Check sheet for the modelled part. Datum: model origin and axes. Units: mm. A direction names the side the tool comes from. Coordinates: 2 decimals unless noted, no trailing zeros. Order: outer loops, then holes, each group sorted by start corner. A loop starts at its lowest first (then second) coordinate and runs counter-clockwise, first axis right, second up.
from build123d import *
from OCP.BRepFilletAPI import BRepFilletAPI_MakeChamfer

# Parameters (mm, degrees)
SCHIZZO1_R                   = 18.5
ESTRUSIONE_ESTRUSIONE1_DEPTH = 29.3
SCHIZZO2_R                   = 16.5
ESTRUSIONE_ESTRUSIONE2_DEPTH = 22.7
SCHIZZO3_R                   = 15.85
TAGLIO_ESTRUSIONE1_DEPTH     = 1.5
SCHIZZO4_R                   = 2.75
SCHIZZO4_R_2                 = 3.925
ESTRUSIONE_ESTRUSIONE3_DEPTH = 2
SCHIZZO5_W                   = 0.5
SCHIZZO5_H                   = 2.9
ESTRUSIONE_ESTRUSIONE4_DEPTH = 4.5
SMUSSO1_SIZE                 = 1
SMUSSO1_SIZE2                = 0.577350269
TAGLIO_ESTRUSIONE2_DEPTH     = 68.129073433
SCHIZZO7_R                   = 1.1
TAGLIO_ESTRUSIONE3_DEPTH     = 2
SCHIZZO8_R                   = 1
ESTRUSIONE_ESTRUSIONE5_DEPTH = 4.75
SCHIZZO9_R                   = 1.5
TAGLIO_ESTRUSIONE4_DEPTH     = 5
SCHIZZO10_R                  = 6
ESTRUSIONE_ESTRUSIONE6_DEPTH = 6
SCHIZZO11_R                  = 3
ESTRUSIONE_ESTRUSIONE7_DEPTH = 3.5
ESTRUSIONE_ESTRUSIONE8_DEPTH = 12
CROQUIS1_R                   = 2
CORTAR_EXTRUIR1_DEPTH        = 10


with BuildPart() as part:
    # Schizzo1 → Estrusione-Estrusione1 (new body)
    with BuildSketch(Plane(origin=(0, 0, 0), x_dir=(1, 0, 0), z_dir=(0, 1, 0))):
        with Locations(Location((0, 0, 0), (0, 0, 270))):
            Circle(SCHIZZO1_R)
    extrude(amount=ESTRUSIONE_ESTRUSIONE1_DEPTH)

    # Schizzo2 → Estrusione-Estrusione2 (add)
    with BuildSketch(Plane(origin=(0, 29.3, 0), x_dir=(1, 0, 0), z_dir=(0, 1, 0))):
        with Locations(Location((0, 0, 0), (0, 0, 270))):
            Circle(SCHIZZO2_R)
    extrude(amount=ESTRUSIONE_ESTRUSIONE2_DEPTH)

    # Schizzo3 → Taglio-Estrusione1 (cut)
    with BuildSketch(Plane(origin=(0, 52, 0), x_dir=(1, 0, 0), z_dir=(0, 1, 0))):
        with Locations(Location((0, 0, 0), (0, 0, 270))):
            Circle(SCHIZZO3_R)
    extrude(amount=-TAGLIO_ESTRUSIONE1_DEPTH, mode=Mode.SUBTRACT)

    # Schizzo4 → Estrusione-Estrusione3 (add)
    with BuildSketch(Plane(origin=(0, 50.5, 0), x_dir=(1, 0, 0), z_dir=(0, 1, 0))):
        with Locations(Location((11.5, 0, 0), (0, 0, 270))):
            Circle(SCHIZZO4_R)
        with Locations(Location((-11.5, 0, 0), (0, 0, 270))):
            Circle(SCHIZZO4_R)
        with Locations(Location((0, 0, 0), (0, 0, 270))):
            Circle(SCHIZZO4_R_2)
    extrude(amount=ESTRUSIONE_ESTRUSIONE3_DEPTH)

    # Schizzo5 → Estrusione-Estrusione4 (add)
    with BuildSketch(Plane(origin=(0, 52.5, 0), x_dir=(1, 0, 0), z_dir=(0, 1, 0))):
        with Locations((-11.5, 0)):
            Rectangle(SCHIZZO5_W, SCHIZZO5_H)
        with Locations((11.5, 0)):
            Rectangle(SCHIZZO5_W, SCHIZZO5_H)
    extrude(amount=ESTRUSIONE_ESTRUSIONE4_DEPTH)

    # Smusso1: one chamfer whose edges measure the first distance from different faces: ONE call of the kernel's chamfer builder (chamfer() names one face for all edges)
    smusso1_edges_1 = [part.edges().sort_by_distance(p)[0] for p in [
        (-11.5, 57, -1.45),
    ]]
    smusso1_side_1 = [part.faces().sort_by_distance(p)[0] for p in [
        (-11.5, 54.75, -1.45),
    ]]
    smusso1_edges_2 = [part.edges().sort_by_distance(p)[0] for p in [
        (-11.5, 57, 1.45),
    ]]
    smusso1_side_2 = [part.faces().sort_by_distance(p)[0] for p in [
        (-11.5, 54.75, 1.45),
    ]]
    smusso1_edges_3 = [part.edges().sort_by_distance(p)[0] for p in [
        (11.5, 57, -1.45),
    ]]
    smusso1_side_3 = [part.faces().sort_by_distance(p)[0] for p in [
        (11.5, 54.75, -1.45),
    ]]
    smusso1_edges_4 = [part.edges().sort_by_distance(p)[0] for p in [
        (11.5, 57, 1.45),
    ]]
    smusso1_side_4 = [part.faces().sort_by_distance(p)[0] for p in [
        (11.5, 54.75, 1.45),
    ]]
    smusso1 = BRepFilletAPI_MakeChamfer(part.part.solid().wrapped)
    for e in smusso1_edges_1:
        smusso1.Add(SMUSSO1_SIZE, SMUSSO1_SIZE2, e.wrapped, smusso1_side_1[0].wrapped)  # the first distance lies on this face
    for e in smusso1_edges_2:
        smusso1.Add(SMUSSO1_SIZE, SMUSSO1_SIZE2, e.wrapped, smusso1_side_2[0].wrapped)  # the first distance lies on this face
    for e in smusso1_edges_3:
        smusso1.Add(SMUSSO1_SIZE, SMUSSO1_SIZE2, e.wrapped, smusso1_side_3[0].wrapped)  # the first distance lies on this face
    for e in smusso1_edges_4:
        smusso1.Add(SMUSSO1_SIZE, SMUSSO1_SIZE2, e.wrapped, smusso1_side_4[0].wrapped)  # the first distance lies on this face
    add(Compound.cast(smusso1.Shape()), mode=Mode.REPLACE)

    # Schizzo6 → Taglio-Estrusione2 (cut, through all)
    with BuildSketch(Plane.ZY.offset(11.75)):
        with BuildLine():
            Line((0.675, 55.35), (0.675, 53.35))
            ThreePointArc((0.675, 53.35), (0, 52.675), (-0.675, 53.35))
            Line((-0.675, 53.35), (-0.675, 55.35))
            ThreePointArc((-0.675, 55.35), (0, 56.025), (0.675, 55.35))
        make_face()
    extrude(amount=-TAGLIO_ESTRUSIONE2_DEPTH, mode=Mode.SUBTRACT)

    # Schizzo7 → Taglio-Estrusione3 (cut)
    with BuildSketch(Plane(origin=(0, 52.5, 0), x_dir=(1, 0, 0), z_dir=(0, 1, 0))):
        with Locations(Location((0, 0, 0), (0, 0, 270))):
            Circle(SCHIZZO7_R)
    extrude(amount=-TAGLIO_ESTRUSIONE3_DEPTH, mode=Mode.SUBTRACT)

    # Schizzo8 → Estrusione-Estrusione5 (add)
    with BuildSketch(Plane(origin=(0, 50.5, 0), x_dir=(1, 0, 0), z_dir=(0, 1, 0))):
        with Locations(Location((0, 0, 0), (0, 0, 270))):
            Circle(SCHIZZO8_R)
    extrude(amount=ESTRUSIONE_ESTRUSIONE5_DEPTH)

    # Schizzo9 → Taglio-Estrusione4 (cut)
    with BuildSketch(Plane.XZ):
        with Locations(Location((0, -15.5, 0), (0, 0, 270))):
            Circle(SCHIZZO9_R)
        with Locations(Location((-13.423393759, -7.75, 0), (0, 0, 270))):
            Circle(SCHIZZO9_R)
        with Locations(Location((-13.423393759, 7.75, 0), (0, 0, 270))):
            Circle(SCHIZZO9_R)
        with Locations(Location((0, 15.5, 0), (0, 0, 270))):
            Circle(SCHIZZO9_R)
        with Locations(Location((13.423393759, 7.75, 0), (0, 0, 270))):
            Circle(SCHIZZO9_R)
        with Locations(Location((13.423393759, -7.75, 0), (0, 0, 270))):
            Circle(SCHIZZO9_R)
    extrude(amount=-TAGLIO_ESTRUSIONE4_DEPTH, mode=Mode.SUBTRACT)

    # Schizzo10 → Estrusione-Estrusione6 (add)
    with BuildSketch(Plane.XZ):
        with Locations(Location((-6.5, 0, 0), (0, 0, 270))):
            Circle(SCHIZZO10_R)
    extrude(amount=ESTRUSIONE_ESTRUSIONE6_DEPTH)

    # Schizzo11 → Estrusione-Estrusione7 (add)
    with BuildSketch(Plane.XZ.offset(6)):
        with Locations(Location((-6.5, 0, 0), (0, 0, 270))):
            Circle(SCHIZZO11_R)
    extrude(amount=ESTRUSIONE_ESTRUSIONE7_DEPTH)

    # Schizzo12 → Estrusione-Estrusione8 (add)
    with BuildSketch(Plane.XZ.offset(9.5)):
        with BuildLine():
            ThreePointArc((-9.5, 0), (-7.448683298, -2.846049894), (-4.1, -1.8))
            Line((-4.1, -1.8), (-4.1, 0))
            Line((-4.1, 0), (-9.5, 0))
        make_face()
        with BuildLine():
            Line((-9.5, 0), (-4.1, 0))
            Line((-4.1, 0), (-4.1, 1.8))
            ThreePointArc((-4.1, 1.8), (-7.448683298, 2.846049894), (-9.5, 0))
        make_face()
    extrude(amount=ESTRUSIONE_ESTRUSIONE8_DEPTH)

    # Croquis1 → Cortar-Extruir1 (cut)
    with BuildSketch(Plane.XZ):
        with Locations(Location((7.75, -13.423393759, 0), (0, 0, 270))):
            Circle(CROQUIS1_R)
        with Locations(Location((-15.5, 0, 0), (0, 0, 270))):
            Circle(CROQUIS1_R)
        with Locations(Location((7.75, 13.423393759, 0), (0, 0, 270))):
            Circle(CROQUIS1_R)
    extrude(amount=-CORTAR_EXTRUIR1_DEPTH, mode=Mode.SUBTRACT)


solid = part.part
(1) Cross-section at D-D (y = 39). Enter the section's corners in (x, z).
Filled in:
outline: circle Ø33 at (0, 0)
(2) Go/stop test with flat-tipped pins: P1, Ø8.5, axis at x = 1.5, z = -1.5, coming from the +Y side; P2, Ø5, axis at y = 38, z = 2.5, coming from the -X side; P3, Ø4.5, axis at x = -15.5, z = 0, coming from the -Y side. Record where each tip stops, or that it passes through.
Filled in:
P1: stops at y = 55.25
P2: stops at x = -16.5
P3: stops at y = 0
(3) Cross-section at B-B (y = 19). Enter the section's corners in (x, z).
Filled in:
outline: circle Ø37 at (0, 0)
(4) Cross-section at C-C (x = -6.5). Enter the section's corners in (y, z).
Filled in:
outline: (-21.5, -3) - (-6, -3) - (-6, -6) - (0, -6) - (0, -17.32) - (29.3, -17.32) - (29.3, -15.17) - (52, -15.17) - (52, -14.46) - (50.5, -14.46) - (50.5, 14.46) - (52, 14.46) - (52, 15.17) - (29.3, 15.17) - (29.3, 17.32) - (0, 17.32) - (0, 6) - (-6, 6) - (-6, 3) - (-21.5, 3) - close
(5) Release check for a two-part mould opening along X. For faces 4 (the flat face through (-11.75, 55, 1)), 5 (the flat face through (-13, 5, 8)), 6 (the cylindrical face through (-16.108, 40.491, -3.577)) record: +X half, -X half, draft (parallel to the pull), parting line (faces both ways), or undercut.
Filled in:
face 4: -X half
face 5: undercut
face 6: parting line
(6) Cross-section at A-A (z = -7.5). Enter the section's corners in (x, y), and give its area (3 significant figures).
Filled in:
outline: (-16.91, 0) - (-14.9, 0) - (-14.9, 5) - (-11.94, 5) - (-11.94, 0) - (11.94, 0) - (11.94, 5) - (14.9, 5) - (14.9, 0) - (16.91, 0) - (16.91, 29.3) - (14.7, 29.3) - (14.7, 52) - (13.96, 52) - (13.96, 50.5) - (-13.96, 50.5) - (-13.96, 52) - (-14.7, 52) - (-14.7, 29.3) - (-16.91, 29.3) - close
area: 1,590 mm2
(7) Thickness scan on probe 1 along Z at (x, y) = (14, 0.5); probe 2 along Y at (x, z) = (8, 6); probe 3 along Y at (x, z) = (7, 17). Record the ranges inside material, lowest first.
Filled in:
probe 1: z = -12.09 to -9.13, -6.37 to 6.37, 9.13 to 12.09
probe 2: y = 0 to 50.5
probe 3: y = 0 to 29.3
(8) Tool access check on faces 1 (the cylindrical face through (-2.388, 51.486, -3.115)), 2 (the flat face through (-15, 10, 0)), 3 (the flat face through (-11.25, 55, 1)). Record the directions out of +Z, -Z, +X, -X, +Y, -Y that give a thin tool (end or side, any length) a straight path to the whole face; none if there is none.
Filled in:
face 1: +Y
face 2: -Y
face 3: +Z, -Z, +Y
